Read the model definition and answer for the solid it produces. Units are mm, in the model's axes. Coordinates: 2 decimals unless noted, no trailing zeros. Order: outer loops, then holes, each group sorted by start corner. A loop starts at its lowest first (then second) coordinate and runs counter-clockwise, first axis right, second up. Notation, with made-up numbers: M 3.25,41 L 13.25,41 A17 cw 13.25,59 Z; hole C 10.5,75 d9. An arc over 180 degrees is marked long. Put each result on its own line as item: value.
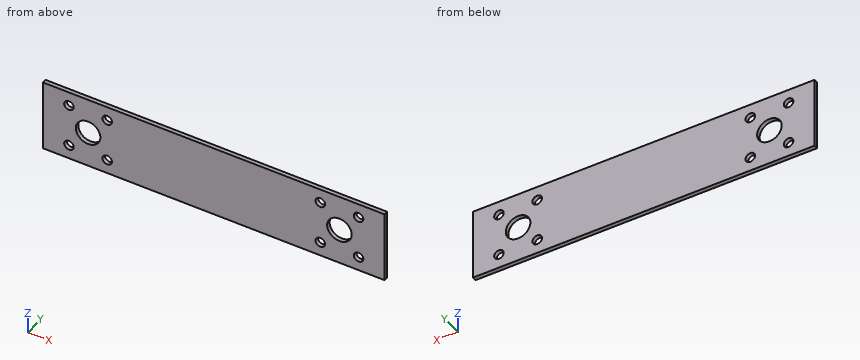
from build123d import *

# Parameters (mm, degrees)
SKETCH4_R           = 1.75
SKETCH4_R_2         = 4.5
BOSS_EXTRUDE1_DEPTH = 1.5


with BuildPart() as part:
    # Sketch4 → Boss-Extrude1 (new body)
    with BuildSketch(Plane(origin=(0, 0, 0), x_dir=(1, 0, 0), z_dir=(0, 1, 0))):
        Polygon((-30.158983798, 50.908297492), (-63.158983798, 50.908297492), (-63.158983798, 24.408297492), (-30.158983798, 24.408297492), (28.841016202, 24.408297492), (61.841016202, 24.408297492), (61.841016202, 50.908297492), (28.841016202, 50.908297492), align=None)
        with Locations(Location((-53.658983798, 29.658297492, 0), (0, 0, 270))):
            Circle(SKETCH4_R, mode=Mode.SUBTRACT)
        with Locations(Location((-39.658983798, 29.658297492, 0), (0, 0, 270))):
            Circle(SKETCH4_R, mode=Mode.SUBTRACT)
        with Locations(Location((38.341016202, 29.658297492, 0), (0, 0, 270))):
            Circle(SKETCH4_R, mode=Mode.SUBTRACT)
        with Locations(Location((52.341016202, 29.658297492, 0), (0, 0, 270))):
            Circle(SKETCH4_R, mode=Mode.SUBTRACT)
        with Locations(Location((-46.658983798, 37.658297492, 0), (0, 0, 270))):
            Circle(SKETCH4_R_2, mode=Mode.SUBTRACT)
        with Locations(Location((-53.658983798, 45.658297492, 0), (0, 0, 270))):
            Circle(SKETCH4_R, mode=Mode.SUBTRACT)
        with Locations(Location((-39.658983798, 45.658297492, 0), (0, 0, 270))):
            Circle(SKETCH4_R, mode=Mode.SUBTRACT)
        with Locations(Location((45.341016202, 37.658297492, 0), (0, 0, 270))):
            Circle(SKETCH4_R_2, mode=Mode.SUBTRACT)
        with Locations(Location((38.341016202, 45.658297492, 0), (0, 0, 270))):
            Circle(SKETCH4_R, mode=Mode.SUBTRACT)
        with Locations(Location((52.341016202, 45.658297492, 0), (0, 0, 270))):
            Circle(SKETCH4_R, mode=Mode.SUBTRACT)
    extrude(amount=BOSS_EXTRUDE1_DEPTH)


solid = part.part
Q1. Find section B-B on z = -40.25. Write down the section's boundary in (x, y), plus the area to 3 significant figures.
Answers below:
outline: M -63.16,0 L -50.34,0 L -50.34,1.5 L -63.16,1.5 Z; M -42.98,0 L 41.66,0 L 41.66,1.5 L -42.98,1.5 Z; M 49.02,0 L 61.84,0 L 61.84,1.5 L 49.02,1.5 Z
area: 165 mm^2
Q2. Find section D-D on y = 1.1. Give the number of separate pieces and of enclosed holes in the cut face, plus the area to 3 significant figures.
Answers below:
separate pieces: 1
enclosed holes: 10
area: 3,110 mm^2
Q3. Given pin 1 (3 mm diameter, centred on x = -39.66, z = -45.66, fed in from +Y), flat-ended and moving along its own axis, determine where the tip first touches the part or whether it passes through.
Answers below:
pin 1: passes through
Q4. Find section C-C on x = 43.5. Write down the section's boundary in (y, z).
Answers below:
outline: M 0,-50.91 L 1.5,-50.91 L 1.5,-41.76 L 0,-41.76 Z; M 0,-33.55 L 1.5,-33.55 L 1.5,-24.41 L 0,-24.41 Z
Q5. Find section A-A on z = -30. Write down the section's boundary in (x, y), plus the area to 3 significant figures.
Answers below:
outline: M -63.16,0 L -55.38,0 L -55.38,1.5 L -63.16,1.5 Z; M -51.94,0 L -41.38,0 L -41.38,1.5 L -51.94,1.5 Z; M -37.94,0 L 36.62,0 L 36.62,1.5 L -37.94,1.5 Z; M 40.06,0 L 50.62,0 L 50.62,1.5 L 40.06,1.5 Z; M 54.06,0 L 61.84,0 L 61.84,1.5 L 54.06,1.5 Z
area: 167 mm^2
Q6. Consider line 1 along X through (y, z) = (0.2, -37.75); line 2 along X through (y, z) = (1.15, -28.75); line 3 along X through (y, z) = (0.55, -36.5). Determine where each line is inside the solid, lowest interval first.
Answers below:
line 1: x = -63.16 to -51.16, -42.16 to 40.84, 49.84 to 61.84
line 2: x = -63.16 to -55.15, -52.16 to -41.15, -38.16 to 36.85, 39.84 to 50.85, 53.84 to 61.84
line 3: x = -63.16 to -51.01, -42.31 to 40.99, 49.69 to 61.84
